Could you check a few things on this model? Use its own coordinates, in mm. A direction names the side the tool comes from. Give positions to 0.01 mm unless a question says otherwise; leave off trailing zeros. Loops run counter-clockwise (first coordinate to the right, second up) from the corner with the lowest first, then second, coordinate; pieces in that order, holes last. Notation, with made-up numbers: (-34.5, 6.5) -> (11.5, 6.5) arc R18 ccw to (11.5, 23.5) -> close; hole circle Ø8 at (54, 53). An arc over 180 degrees is marked (long way). Put each result on its own line as item: value.
```python
from build123d import *

# Parameters (mm, degrees)
SKETCH2_R               = 46
SKETCH2_R_2             = 18
BOSS_EXTRUDE2_DEPTH     = 5
SKETCH4_R               = 30
SKETCH4_R_2             = 18
BOSS_EXTRUDE3_DEPTH     = 4
SKETCH5_R               = 1.5
CUT_EXTRUDE1_DEPTH      = 66.673434507
CUT_EXTRUDE1_DEPTH_BACK = 66.673434507
REVOLVE1_ANGLE          = 16
CIRPATTERN1_COUNT       = 6


with BuildPart() as part:
    # Sketch2 → Boss-Extrude2 (new body)
    with BuildSketch(Plane.XY):
        Circle(SKETCH2_R)
        Circle(SKETCH2_R_2, mode=Mode.SUBTRACT)
    extrude(amount=BOSS_EXTRUDE2_DEPTH)

    # Sketch4 → Boss-Extrude3 (add)
    with BuildSketch(Plane.XY.offset(5)):
        Circle(SKETCH4_R)
        Circle(SKETCH4_R_2, mode=Mode.SUBTRACT)
    extrude(amount=BOSS_EXTRUDE3_DEPTH)

    # Sketch5 → Cut-Extrude1 (cut, two sides)
    with BuildSketch(Plane(origin=(0, 0, 0), x_dir=(-1, 0, 0), z_dir=(0, 0, -1))) as cut_extrude1_sk:
        with Locations((0, 22)):
            Circle(SKETCH5_R)
        with Locations((19.052558883, -11)):
            Circle(SKETCH5_R)
        with Locations((-19.052558883, -11)):
            Circle(SKETCH5_R)
    extrude(amount=CUT_EXTRUDE1_DEPTH, mode=Mode.SUBTRACT)
    extrude(cut_extrude1_sk.sketch, amount=-CUT_EXTRUDE1_DEPTH_BACK, mode=Mode.SUBTRACT)

    # Sketch6 → Revolve1 (revolve, symmetric)
    with BuildSketch(Plane(origin=(0, 0, 0), x_dir=(0, 0, -1), z_dir=(1, 0, 0))) as revolve1_sk:
        Polygon((-5, 30), (-9, 30), (-5, 46), align=None)
    revolve1 = revolve(axis=Axis((0, 0, 0), (0, 0, -1)), revolution_arc=REVOLVE1_ANGLE / 2)
    revolve1 = revolve1 + revolve(revolve1_sk.sketch, axis=Axis((0, 0, 0), (0, 0, 1)), revolution_arc=REVOLVE1_ANGLE / 2)

    # CirPattern1: Revolve1 ×6 about axis
    cirpattern1_axis = Axis((0, 0, 0), (0, 0, 1))
    for i in range(1, CIRPATTERN1_COUNT):
        add(revolve1.rotate(cirpattern1_axis, i * 360 / CIRPATTERN1_COUNT))


solid = part.part
```
1. If we section it at A-A (y = 0): List the corners of the cut face in (x, z) for me.
Recorded:
outline: (-46, 0) -> (-18, 0) -> (-18, 9) -> (-30, 9) -> (-30, 5) -> (-46, 5) -> close; (18, 0) -> (46, 0) -> (46, 5) -> (30, 5) -> (30, 9) -> (18, 9) -> close
2. I need wall thicknesses on line 1 (Y direction, x = 0, z = 4.5); line 2 (Y direction, x = -6, z = 8); line 3 (Z direction, x = 33, y = 3). Which ranges of each line are inside material? Lowest first, please.
Recorded:
line 1: y = -46 to -18, 18 to 20.5, 23.5 to 46
line 2: y = -29.39 to -16.97, 16.97 to 29.39
line 3: z = 0 to 5
3. I'm going to push flat-ended pins straight in: pin 1 (1.5 mm diameter, centred on y = 19, z = 4, fed in from -X); pin 2 (3.5 mm diameter, centred on x = -19.05, y = -11, fed in from -Z); pin 3 (2 mm diameter, centred on x = 34, y = 8, fed in from +Z); pin 4 (1.5 mm diameter, centred on x = -24.5, z = 5, fed in from -Y). Where does each tip first touch, or does it pass through?
Recorded:
pin 1: stops at x = -42.22
pin 2: stops at z = 0
pin 3: stops at z = 5
pin 4: stops at y = -39.39
4. Thinking about a two-plate mould opening in Y: for faces 5 (the face through (-27.231, -21.275, 6.083)), 6 (the face through (0, 38, 7)), 7 (the face through (-30, 0, 7)), which applies, pulls with the +Y half, pulls with the -Y half, needs draft (parallel to the pull), parting line crosses it, or undercut?
Recorded:
face 5: pulls with the -Y half
face 6: pulls with the +Y half
face 7: undercut
5. If we section it at B-B (x = 0): List the corners of the cut face in (y, z) for me, then the cut area to 3 significant figures.
Recorded:
outline: (-46, 0) -> (-18, 0) -> (-18, 9) -> (-30, 9) -> (-46, 5) -> close; (18, 0) -> (20.5, 0) -> (20.5, 9) -> (18, 9) -> close; (23.5, 0) -> (46, 0) -> (46, 5) -> (30, 9) -> (23.5, 9) -> close
area: 413 mm^2
6. If we section it at C-C (z = 2): List the corners of the cut face in (x, y) for me, then the cut area to 3 significant figures.
Recorded:
outline: circle Ø92 at (0, 0); hole circle Ø3 at (-19.05, -11); hole circle Ø36 at (0, 0); hole circle Ø3 at (0, 22); hole circle Ø3 at (19.05, -11)
area: 5,610 mm^2
7. If we section it at D-D (z = 6.75): List the corners of the cut face in (x, y) for me, then the cut area to 3 significant figures.
Recorded:
outline: (-36.16, -14.61) arc R39 ccw to (-30.73, -24.01) -> (-23.64, -18.47) arc R30 ccw to (-4.18, -29.71) -> (-5.43, -38.62) arc R39 ccw to (5.43, -38.62) -> (4.18, -29.71) arc R30 ccw to (23.64, -18.47) -> (30.73, -24.01) arc R39 ccw to (36.16, -14.61) -> (27.82, -11.24) arc R30 ccw to (27.82, 11.24) -> (36.16, 14.61) arc R39 ccw to (30.73, 24.01) -> (23.64, 18.47) arc R30 ccw to (4.18, 29.71) -> (5.43, 38.62) arc R39 ccw to (-5.43, 38.62) -> (-4.18, 29.71) arc R30 ccw to (-23.64, 18.47) -> (-30.73, 24.01) arc R39 ccw to (-36.16, 14.61) -> (-27.82, 11.24) arc R30 ccw to (-27.82, -11.24) -> close; hole circle Ø3 at (-19.05, -11); hole circle Ø36 at (0, 0); hole circle Ø3 at (0, 22); hole circle Ø3 at (19.05, -11)
area: 2,310 mm^2
8. For faces 1 (the face through (-27.231, 21.275, 6.083)), 2 (the face through (32.04, 12.945, 6.083)), 3 (the face through (32.97, 19.12, 6.97)), 4 (the face through (-32.04, -12.945, 6.083)), which set-ups out of +Z, -Z, +X, -X, +Y, -Y let a thin tool reach every point of the face, with its end or its side?
Recorded:
face 1: +Z, +Y
face 2: +Z, +X
face 3: +Z, +X, +Y
face 4: +Z, -X
